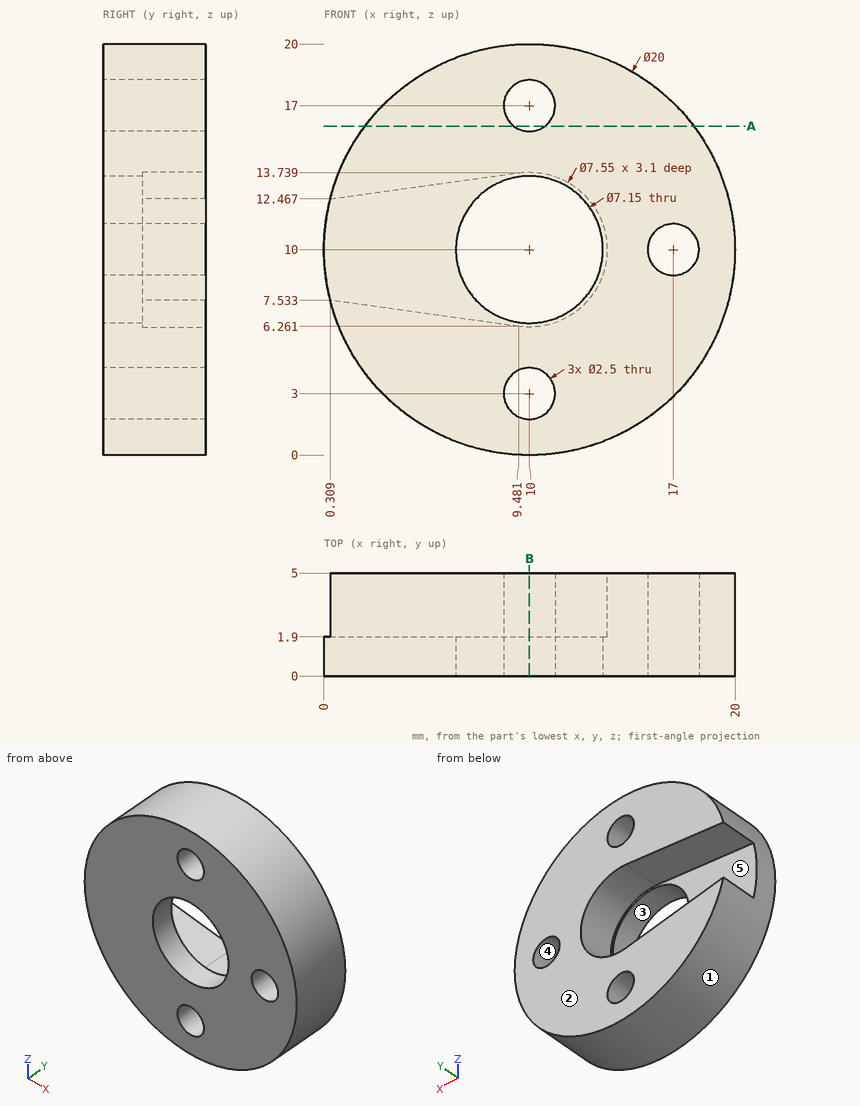
Geometry: see drawing. Coordinates: mm, zero at the bounding-box minimum. A direction names the side the tool comes from. Coordinates: 2 decimals unless noted, no trailing zeros. Loops run counter-clockwise (first coordinate to the right, second up) from the corner with the lowest first, then second, coordinate; pieces in that order, holes last.
(1) Pull-direction query (Z, two-part tool) for the marked faces 1, 2 and 3; classes: released by +Z, released by -Z, zero draft, split by the parting line, or undercut.
(2) First-contact query: pin 1 Ø10 at (x, z) = (10, 10) entering from +Y; pin 2 Ø1 at (y, z) = (4, 3.5) entering from -X. Flat tips, straight axial feed; report the tip coordinate or a pass-through.
(3) Set-up query: the marked faces 4 and 5. Return all of +Z, -Z, +X, -X, +Y, -Y with unobstructed straight access to the full face (end or side cutting, diameter ignored); none if empty.
(4) Material intervals for probe 1 along X at (y, z) = (1.6, 3); probe 2 along Z at (x, y) = (1, 4.75) (1 decimal); probe 3 along Z at (x, y) = (5.5, 2.95), sorted ascending.
(5) Section A-A on z = 16. Return the cut outline in (x, y), then the cut area to 3 significant figures.
(6) Section B-B on x = 10. Count the separate pieces of the cut face and the enclosed holes in it.
Data:
1. face 1: split by the parting line
1. face 2: zero draft
1. face 3: undercut
2. pin 1: stops at y = 5
2. pin 2: stops at x = 2
3. face 4: +Y, -Y
3. face 5: +Y
4. probe 1: x = 2.86 to 8.75, 11.25 to 17.14
4. probe 2: z = 5.6 to 7.4, 12.6 to 14.4
4. probe 3: z = 1.07 to 6.81, 13.19 to 18.93
5. outline: (2, 0) - (9.25, 0) - (9.25, 5) - (2, 5) - close; (10.75, 0) - (18, 0) - (18, 5) - (10.75, 5) - close
5. area: 72.5 mm2
6. separate pieces: 4
6. enclosed holes: 0
